Check sheet for the modelled part. Datum: model origin and axes. Units: mm. Face numbers are marked on the shaded views. Coordinates: 2 decimals unless noted, no trailing zeros. Loops run counter-clockwise (first coordinate to the right, second up) from the corner with the lowest first, then second, coordinate; pieces in that order, holes last. Notation, with made-up numbers: M -21.75,49 L 20.25,49 A11 cw 20.25,57 Z; hole C -18.5,65 d3. An arc over 180 degrees is marked long. Answer in a Markdown table with one row per item. Add a question column.
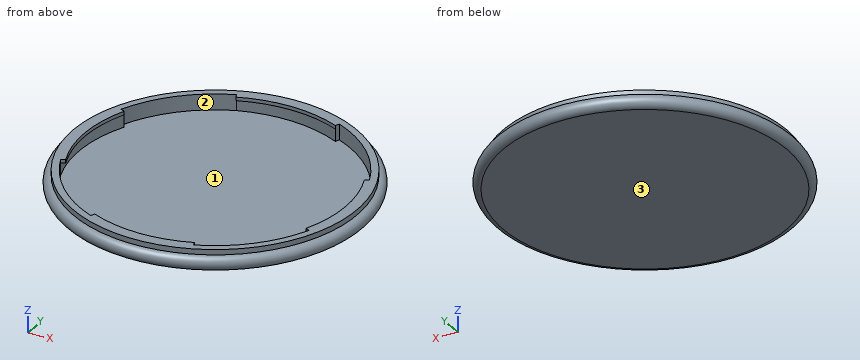
```python
from build123d import *

# Parameters (mm, degrees)
PAD001_DEPTH = 1
PAD_DEPTH    = 5.5


with BuildPart() as part:
    # Sketch (on XZ_Plane of Origin) → Revolution (revolve)
    with BuildSketch(Plane.XZ):
        with BuildLine():
            Line((0, 0), (0, 1))
            Line((0, 1), (-38.5, 1))
            Line((-38.5, 1), (-38.5, 5.5))
            Line((-38.5, 5.5), (-40.5, 5.5))
            Line((-40.5, 5.5), (-40.5, 4))
            ThreePointArc((-40.5, 4), (-42.5, 2), (-40.5, 0))
            Line((0, 0), (-40.5, 0))
        make_face()
    revolve(axis=Axis((0, 0, 0), (0, 0, 1)))

    # Sketch001 (on Face3 of Revolution) → Pad001 (new body)
    with BuildSketch(Plane.XY.offset(5.5)):
        with BuildLine():
            ThreePointArc((14.733312, 35.569362), (0, 38.5), (-14.733312, 35.569362))
            Line((-14.254958, 34.414513), (-14.733312, 35.569362))
            ThreePointArc((14.254958, 34.414513), (0, 37.25), (-14.254958, 34.414513))
            Line((14.254958, 34.414513), (14.733312, 35.569362))
        make_face()
        with BuildLine():
            ThreePointArc((34.414513, -14.254958), (37.25, 0), (34.414513, 14.254958))
            Line((34.414513, 14.254958), (35.569362, 14.733312))
            ThreePointArc((35.569362, -14.733312), (38.5, 0), (35.569362, 14.733312))
            Line((34.414513, -14.254958), (35.569362, -14.733312))
        make_face()
        with BuildLine():
            ThreePointArc((-14.254958, -34.414513), (0, -37.25), (14.254958, -34.414513))
            Line((14.254958, -34.414513), (14.733312, -35.569362))
            ThreePointArc((-14.733312, -35.569362), (0, -38.5), (14.733312, -35.569362))
            Line((-14.733312, -35.569362), (-14.254958, -34.414513))
        make_face()
        with BuildLine():
            ThreePointArc((-34.414513, 14.254958), (-37.25, 0), (-34.414513, -14.254958))
            Line((-34.414513, -14.254958), (-35.569362, -14.733312))
            ThreePointArc((-35.569362, 14.733312), (-38.5, 0), (-35.569362, -14.733312))
            Line((-35.569362, 14.733312), (-34.414513, 14.254958))
        make_face()
    extrude(amount=-PAD001_DEPTH)

    # Sketch002 (on Face4 of Pad001) → Pad (join)
    with BuildSketch(Plane.XY.offset(5.5)):
        with BuildLine():
            Line((-35.569362, 14.733312), (-34.414513, 14.254958))
            ThreePointArc((-34.414513, 14.254958), (-37.875, -0.12432), (-35.569362, -14.733312))
            ThreePointArc((-35.569362, 14.733312), (-38.5, 0), (-35.569362, -14.733312))
        make_face()
        with BuildLine():
            ThreePointArc((14.733312, 35.569362), (0, 38.5), (-14.733312, 35.569362))
            ThreePointArc((14.254958, 34.414513), (-0.12432, 37.875), (-14.733312, 35.569362))
            Line((14.733312, 35.569362), (14.254958, 34.414513))
        make_face()
        with BuildLine():
            ThreePointArc((35.569362, -14.733312), (38.5, 0), (35.569362, 14.733312))
            ThreePointArc((34.414513, -14.254958), (37.875, 0.12432), (35.569362, 14.733312))
            Line((35.569362, -14.733312), (34.414513, -14.254958))
        make_face()
        with BuildLine():
            ThreePointArc((-14.733312, -35.569362), (0, -38.5), (14.733312, -35.569362))
            ThreePointArc((-14.254958, -34.414513), (0.12432, -37.875), (14.733312, -35.569362))
            Line((-14.733312, -35.569362), (-14.254958, -34.414513))
        make_face()
    extrude(amount=-PAD_DEPTH)


solid = part.part
```
Q1. Mould release check, pull along X, two halves, no side actions. Record for the marked faces 1, 2 and 3: released by +X, released by -X, zero draft, split by the parting line, or undercut.
Q2. Cross-section at B-B (x = 0). Record the cut outline in (y, z), plus the area to 3 significant figures.
Q3. Go/stop test with flat-tipped pins: pin 1 (5 mm diameter, centred on x = -8, y = 24.5, fed in from +Z); pin 2 (1 mm diameter, centred on x = 1.5, z = 3.5, fed in from -Y). Record where each tip stops, or that it passes through.
Q4. Thickness scan on L1, parallel to Z at x = -29.5, y = 24.5; L2, parallel to Y at x = -15, z = 2.8; L3, parallel to X at y = 8, z = 3.2. Record the ranges inside material, lowest first.
Q5. Cross-section at A-A (z = 2.7). Record the cut outline in (x, y), plus the area to 3 significant figures.
Answer key:
| question | item | result |
|---|---|---|
| 1 | face 1 | undercut |
| 1 | face 2 | undercut |
| 1 | face 3 | zero draft |
| 2 | outline | M -40.5,0 L 40.5,0 A2 ccw 40.5,4 L 40.5,5.5 L 37.25,5.5 L 37.25,4.5 L 37.87,4.5 L 37.87,1 L -37.87,1 L -37.87,4.5 L -37.25,4.5 L -37.25,5.5 L -40.5,5.5 L -40.5,4 A2 ccw Z |
| 2 | area | 118 mm^2 |
| 3 | pin 1 | z = 1 |
| 3 | pin 2 | y = -42.21 |
| 4 | L1 | 0 to 1 |
| 4 | L2 | -39.59 to -35.46, 35.46 to 39.59 |
| 4 | L3 | -41.33 to -36.66, 37.37 to 41.33 |
| 5 | outline | C 0,0 d84.75; hole M -35.57,-14.73 A38.5 ccw -14.73,-35.57 L -14.25,-34.41 A37.91 ccw 14.73,-35.57 A38.5 ccw 35.57,-14.73 L 34.41,-14.25 A37.91 ccw 35.57,14.73 A38.5 ccw 14.73,35.57 L 14.25,34.41 A37.91 ccw -14.73,35.57 A38.5 ccw -35.57,14.73 L -34.41,14.25 A37.91 ccw Z |
| 5 | area | 1,060 mm^2 |
